Check sheet for the modelled part. Datum: model origin and axes. Units: mm. Give positions to 0.01 mm unless a question says otherwise; leave off trailing zeros. Order: outer loops, then holes, each group sorted by start corner. A loop starts at its lowest first (then second) coordinate and runs counter-clockwise, first axis right, second up. Notation, with made-up numbers: (-23, 24.5) -> (-13, 24.5) arc R18 ccw to (-13, 52.5) -> close; hole circle Ø7 at (-18, 3.5). An arc over 180 degrees is marked (long way). One line per question, with ' | ' between items.
```python
from build123d import *

# Parameters (mm, degrees)
SKETCH1_R           = 76.073
SKETCH1_R_2         = 4.8641
BOSS_EXTRUDE1_DEPTH = 12.7
SKETCH2_W           = 6.1976
SKETCH2_H           = 12.2682
CUT_EXTRUDE1_DEPTH  = 109.330478897
SKETCH3_R           = 11.303
CUT_EXTRUDE2_DEPTH  = 7.62
CUT_EXTRUDE3_START  = 76.073
SKETCH5_R           = 1.524
CUT_EXTRUDE3_DEPTH  = 6.35
CUT_EXTRUDE4_START  = -69.723
SKETCH6_R           = 1.524
CUT_EXTRUDE4_DEPTH  = 6.35


with BuildPart() as part:
    # Sketch1 → Boss-Extrude1 (new body)
    with BuildSketch(Plane.XY):
        Circle(SKETCH1_R)
        with Locations((0, -6.35)):
            Circle(SKETCH1_R_2, mode=Mode.SUBTRACT)
    extrude(amount=BOSS_EXTRUDE1_DEPTH)

    # Sketch2 → Cut-Extrude1 (cut, through all)
    with BuildSketch(Plane.XY.offset(12.7)):
        with Locations((68.3851714, -10.5537)):
            Rectangle(SKETCH2_W, SKETCH2_H)
        Polygon((-71.4839714, -4.4958), (-71.4839714, -16.6878), (-65.2863714, -16.6878), (-65.2863714, -4.4196), (-66.357360373, -4.4196), (-66.357360373, -4.4958), align=None)
    extrude(amount=-CUT_EXTRUDE1_DEPTH, mode=Mode.SUBTRACT)

    # Sketch3 → Cut-Extrude2 (cut)
    with BuildSketch(Plane.XY.offset(12.7)):
        with Locations((0, -6.35)):
            Circle(SKETCH3_R)
    extrude(amount=-CUT_EXTRUDE2_DEPTH, mode=Mode.SUBTRACT)

    # Sketch5 → Cut-Extrude3 (cut)
    with BuildSketch(Plane(origin=(0, 0, 0), x_dir=(1, 0, 0), z_dir=(0, 1, 0)).offset(CUT_EXTRUDE3_START)):
        with Locations(Location((0, -6.35, 0), (0, 0, 270))):
            Circle(SKETCH5_R)
    extrude(amount=-CUT_EXTRUDE3_DEPTH, mode=Mode.SUBTRACT)

    # Sketch6 → Cut-Extrude4 (cut)
    with BuildSketch(Plane(origin=(0, 0, 0), x_dir=(1, 0, 0), z_dir=(0, 1, 0)).offset(CUT_EXTRUDE4_START)):
        with Locations(Location((0, -6.35, 0), (0, 0, 270))):
            Circle(SKETCH6_R)
    extrude(amount=-CUT_EXTRUDE4_DEPTH, mode=Mode.SUBTRACT)


solid = part.part
```
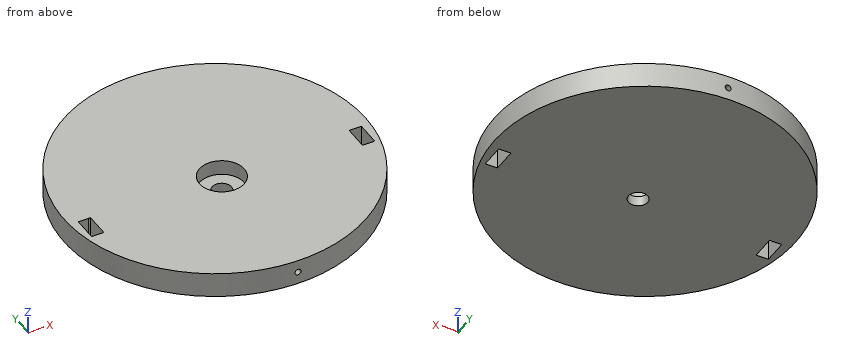
Q1. Thickness scan on line 1 (Z direction, x = 0, y = -72); line 2 (X direction, y = -6.35, z = 3.8); line 3 (Y direction, x = 0, z = 3.45). Record the ranges inside material, lowest first.
Result sheet:
line 1: z = 0 to 4.83, 7.87 to 12.7 | line 2: x = -75.81 to -71.48, -65.29 to -4.86, 4.86 to 65.29, 71.48 to 75.81 | line 3: y = -76.07 to -11.21, -1.49 to 76.07
Q2. Section check C-C (y = -55.5). Enter the section's corners in (x, z), and give its area (3 significant figures).
Result sheet:
outline: (-52.03, 0) -> (52.03, 0) -> (52.03, 12.7) -> (-52.03, 12.7) -> close | area: 1,320 mm2
Q3. Section check B-B (x = -61). Enter the section's corners in (y, z).
Result sheet:
outline: (-45.45, 0) -> (45.45, 0) -> (45.45, 12.7) -> (-45.45, 12.7) -> close
Q4. Depth check by flat-ended pin: pin 1 Ø0.9 at (x, z) = (-66, 8.5) entering from -Y; pin 2 Ø6 at (y, z) = (-9.5, 6.5) entering from +X; pin 3 Ø7 at (x, y) = (2, -11.5) entering from +Z; pin 4 Ø10 at (x, y) = (-60.5, -58.5) entering from -Z. Enter the tip coordinate at first touch or a pass-through.
Result sheet:
pin 1: stops at y = -38.6 | pin 2: stops at x = 75.79 | pin 3: stops at z = 5.08 | pin 4: passes through
Q5. Section check A-A (y = -6.35). Enter the section's corners in (x, z), and give its area (3 significant figures).
Result sheet:
outline: (-75.81, 0) -> (-71.48, 0) -> (-71.48, 12.7) -> (-75.81, 12.7) -> close; (-65.29, 0) -> (-4.86, 0) -> (-4.86, 5.08) -> (-11.3, 5.08) -> (-11.3, 12.7) -> (-65.29, 12.7) -> close; (4.86, 0) -> (65.29, 0) -> (65.29, 12.7) -> (11.3, 12.7) -> (11.3, 5.08) -> (4.86, 5.08) -> close; (71.48, 0) -> (75.81, 0) -> (75.81, 12.7) -> (71.48, 12.7) -> close | area: 1,550 mm2
